Autodesk Inventor part; units mm, degrees
ref_plane "YZ Plane" through (0, 0, 0) normal (1, 0, 0) x (0, 1, 0)
ref_plane "XZ Plane" through (0, 0, 0) normal (0, 1, 0) x (-1, 0, 0)
ref_plane "XY Plane" through (0, 0, 0) normal (0, 0, 1) x (1, 0, 0)
sketch "Sketch1" plane through (0, 0, 0) normal (0, 0, 1) x (1, 0, 0)
  line L0 (-35.9682, 33.3635) -> (34.0318, 33.3635)
  line L1 (-45.9682, -16.6365) -> (-45.9682, 23.3635)
  circle A0 centre (-45.9682, 33.3635) radius 5
  circle A1 centre (44.0318, 33.3635) radius 5
  circle A2 centre (44.0318, -26.6365) radius 5
  circle A3 centre (-45.9682, -26.6365) radius 5
  arc A4 (-35.9682, 33.3635) -> (-45.9682, 23.3635) centre (-45.9682, 33.3635) ccw
  arc A5 (44.0318, 23.3635) -> (34.0318, 33.3635) centre (44.0318, 33.3635) ccw
  arc A6 (34.0318, -26.6365) -> (44.0318, -16.6365) centre (44.0318, -26.6365) ccw
  arc A7 (-45.9682, -16.6365) -> (-35.9682, -26.6365) centre (-45.9682, -26.6365) ccw
  line L2 (34.0318, -26.6365) -> (-35.9682, -26.6365)
  line L3 (44.0318, 23.3635) -> (44.0318, -16.6365)
  arc A8 (-33, 18.7271) -> (-37, 18.7271) centre (-35, 18.7271) ccw
  arc A9 (-37, -12) -> (-33, -12) centre (-35, -12) ccw
  arc A10 (37, 18.7271) -> (33, 18.7271) centre (35, 18.7271) ccw
  arc A11 (33, -12) -> (37, -12) centre (35, -12) ccw
  line L4 (-37, 18.7271) -> (-37, -12)
  line L5 (-33, -12) -> (-33, 18.7271)
  line L6 (33, 18.7271) -> (33, -12)
  line L7 (37, -12) -> (37, 18.7271)
  circle A12 centre (0, 3.3635) radius 10
  circle A13 centre (22.145, 14.9653) radius 2.5
  circle A14 centre (-14.6946, 23.589) radius 2.5
  circle A15 centre (-23.7764, 11.089) radius 2.5
  circle A16 centre (-23.7764, -4.3619) radius 2.5
  circle A17 centre (-14.6946, -16.8619) radius 2.5
  circle A18 centre (0, -21.6365) radius 2.5
  circle A19 centre (0, 28.3635) radius 2.5
  dimension "d22" = 242.35
extrude "Extrusion1" add sketch "Sketch1" along normal blind 3
fillet "Fillet1" radius 3 8 edges at (-35.9682, 33.3635, 1.5) (44.0318, -16.6365, 1.5) (-45.9682, -16.6365, 1.5) (34.0318, 33.3635, 1.5) (34.0318, -26.6365, 1.5) (-45.9682, 23.3635, 1.5) (-35.9682, -26.6365, 1.5) (44.0318, 23.3635, 1.5)
properties part number "Desafio 3 - MASA - Inventor"
The model under review builds one solid part; all positions refer to its coordinate system, in mm. A direction names the side the tool comes from. Give positions to 0.01 mm unless a question says otherwise; leave off trailing zeros. Loops run counter-clockwise (first coordinate to the right, second up) from the corner with the lowest first, then second, coordinate; pieces in that order, holes last. Notation, with made-up numbers: (9.5, 66.25) -> (44.5, 66.25) arc R25 ccw to (44.5, 105.25) -> close; hole circle Ø4 at (54, 80.5). An arc over 180 degrees is marked (long way). Put each result on its own line as item: value. Start each with the question number.
1. Clearance check with flat-ended pins moving along their axes: P1, Ø6.5, axis at x = -23.78, y = -4.36, coming from the +Z side; P2, Ø1, axis at y = -21.5, z = 1, coming from the -X side; P3, Ø1.5, axis at y = -11, z = 0.5, coming from the +X side; P4, Ø1, axis at x = -15.5, z = 2, coming from the -Y side. State where each tip first meets the part, or that it passes through.
2. We need section D-D on z = 1.55. State how many separate pieces and enclosed holes the cut face has, then the cut area to 3 significant figures.
3. We need section B-B on x = 0. State the section outline as (y, z) points.
4. Mouldability with a two-part tool opening along X and no side actions: class faces 1 (the face through (33.22, 33.99, 1.52)), 2 (the face through (-0.325, 25.885, 1.479)), 3 (the face through (-46.597, 22.553, 1.521)), 4 (the face through (-14, 4, 3)) as released by +X, released by -X, zero draft, split by the parting line, or undercut.
5. We need section A-A on y = -9. State the section outline as (x, z) points, then the cut area to 3 significant figures.
6. Wall thickness on probe 1 along X at (y, z) = (18.5, 0.5); probe 2 along Y at (x, z) = (-25.5, 0.4); probe 3 along X at (y, z) = (11, 2.8): over which ranges is each line inside the solid? List them lowest first.
7. We need section C-C on x = -35. State the section outline as (y, z) points, then the cut area to 3 significant figures.
8. For faces 5 (the face through (-37, 4, 1)), 6 (the face through (33.265, -27.301, 1.521)), 7 (the face through (-45.968, 3, 1)), list the 3-axis set-ups (+Z, -Z, +X, -X, +Y, -Y) from which the entire face can be reached by the end or side of a thin tool; tool diameter is ignored.
Determined:
1. P1: z = 3
1. P2: x = -54.83
1. P3: x = 44.03
1. P4: y = -26.64
2. separate pieces: 1
2. enclosed holes: 14
2. area: 5,320 mm^2
3. outline: (-26.64, 0) -> (-24.14, 0) -> (-24.14, 3) -> (-26.64, 3) -> close; (-19.14, 0) -> (-6.64, 0) -> (-6.64, 3) -> (-19.14, 3) -> close; (13.36, 0) -> (25.86, 0) -> (25.86, 3) -> (13.36, 3) -> close; (30.86, 0) -> (33.36, 0) -> (33.36, 3) -> (30.86, 3) -> close
4. face 1: undercut
4. face 2: undercut
4. face 3: released by -X
4. face 4: zero draft
5. outline: (-45.97, 0) -> (-37, 0) -> (-37, 3) -> (-45.97, 3) -> close; (-33, 0) -> (33, 0) -> (33, 3) -> (-33, 3) -> close; (37, 0) -> (44.03, 0) -> (44.03, 3) -> (37, 3) -> close
5. area: 246 mm^2
6. probe 1: -45.97 to -37, -33 to 33, 37 to 44.03
6. probe 2: -26.64 to -6.17, -2.55 to 9.28, 12.9 to 33.36
6. probe 3: -45.97 to -37, -33 to -26.27, -21.28 to -6.46, 6.46 to 33, 37 to 44.03
7. outline: (-27.15, 0) -> (-14, 0) -> (-14, 3) -> (-27.15, 3) -> close; (20.73, 0) -> (33.88, 0) -> (33.88, 3) -> (20.73, 3) -> close
7. area: 78.9 mm^2
8. face 5: +Z, -Z
8. face 6: +Z, -Z, -Y
8. face 7: +Z, -Z, -X
